Solid Edge part; units mm, degrees
sketch "Sketch1" plane through (0, 0, 0) normal (1, 0, 0) x (0, 1, 0)
  line L0 (-108.1482, 2.6153) -> (-28.1482, 2.6153)
  line L1 (-28.1482, 2.6153) -> (-28.1482, 82.6153)
  line L2 (-28.1482, 82.6153) -> (-108.1482, 82.6153)
  line L3 (-108.1482, 82.6153) -> (-108.1482, 2.6153)
  line L4 (-118.1482, -7.3837) -> (-18.1482, -7.3837)
  line L5 (-18.1482, -7.3837) -> (-18.1482, 92.6144)
  line L6 (-18.1482, 92.6144) -> (-118.1482, 92.6163)
  line L7 (-118.1482, 92.6163) -> (-118.1482, -7.3837)
  dimension "D1" = 28.1482
  dimension "D2" = 108.1482
extrude "Protrusion1" add sketch "Sketch1" against normal blind 1850
sketch "Sketch2" plane through (-925, -118.1482, 42.6163) normal (0, -1, 0) x (-1, 0, 0)
  circle A0 centre (-905, -20) radius 4.1
  circle A1 centre (-865, 20) radius 4.1
  circle A2 centre (-865, -20) radius 4.1
  circle A3 centre (-905, 20) radius 4.1
extrude "Cutout1" cut sketch "Sketch2" against normal through all
mirror "Mirror1" about plane through (-925, -153.5035, -42.739) normal (0, 0.7071, -0.7071) of "Cutout1"
sketch "Sketch3" plane through (-925, -68.1482, -7.3837) normal (0, 0, -1) x (1, 0, 0)
  circle A0 centre (-855, -30) radius 4.1
  circle A1 centre (-805, 30) radius 4.1
  circle A2 centre (-805, -30) radius 4.1
  circle A3 centre (-755, 30) radius 4.1
  circle A4 centre (-755, -30) radius 4.1
  circle A5 centre (-855, 30) radius 4.1
extrude "Cutout3" cut sketch "Sketch3" against normal blind 46.6265
properties material "Aluminum, 6061-T6"
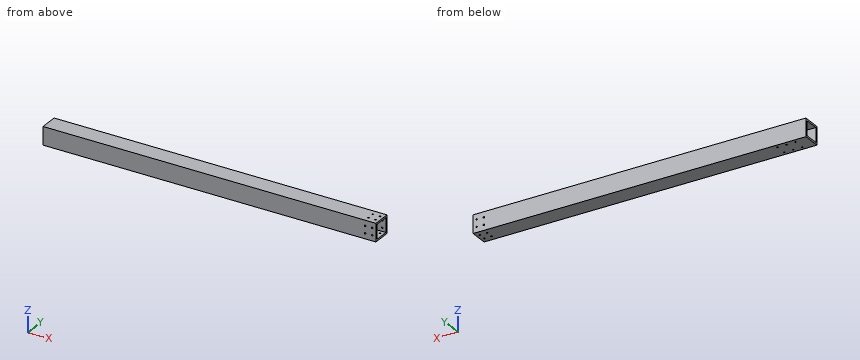
Check sheet for the modelled part. Datum: model origin and axes. Units: mm. Round coordinates to 2 decimals unless told otherwise and drop trailing zeros. Loops run counter-clockwise (first coordinate to the right, second up) from the corner with the lowest first, then second, coordinate; pieces in that order, holes last. Notation, with made-up numbers: (72.25, 36.25) -> (110.25, 36.25) arc R12 ccw to (110.25, 42.25) -> close; hole circle Ø4 at (5, 82). An arc over 180 degrees is marked (long way). Put each result on its own line as item: value. Start each with the question number.
1. Scan lines: probe 1 along Y at (x, z) = (-20, 86); probe 2 along Z at (x, y) = (-60, -115); probe 3 along Y at (x, z) = (-1549, 14.5). Record each from-to range of solid material in increasing order.
2. Gauge pin test, flat end, axial feed: pin 1 (5 mm diameter, centred on x = -20, z = 62.62, fed in from +Y). Record the tip position at first contact, or that the pin passes through.
3. Section check A-A (x = -925.5). Enter the section's corners in (y, z).
Findings:
1. probe 1: y = -118.15 to -92.25, -84.05 to -52.25, -44.05 to -18.15
1. probe 2: z = -7.38 to 18.52, 26.72 to 58.52, 66.72 to 92.62
1. probe 3: y = -118.15 to -108.15, -28.15 to -18.15
2. pin 1: passes through
3. outline: (-118.15, -7.38) -> (-18.15, -7.38) -> (-18.15, 92.61) -> (-118.15, 92.62) -> close; hole (-108.15, 2.62) -> (-28.15, 2.62) -> (-28.15, 82.62) -> (-108.15, 82.62) -> close
